Could you check a few things on this model? Use its own coordinates, in mm. A direction names the side the tool comes from. Round coordinates to 2 decimals unless told otherwise and drop trailing zeros. Loops run counter-clockwise (first coordinate to the right, second up) from the corner with the lowest first, then second, coordinate; pieces in that order, holes last. Notation, with made-up numbers: (42.25, 37.25) -> (55.25, 37.25) arc R29 cw to (55.25, 57.25) -> close; hole circle Ø2 at (66, 48.5). An arc over 180 degrees is marked (long way). One line per item, written item: value.
```python
from build123d import *

# Parameters (mm, degrees)
F1_DEPTH     = 3
F3_D         = 7
F4_W         = 24
F4_H         = 18
F5_DEPTH     = 27
F6_R         = 1.55
F7_DEPTH     = 12.5
F8_R         = 1.75
F9_DEPTH     = 12
F10_R        = 4
F11_DEPTH    = 3.4
F12_T4_DEPTH = 62
F12_T9_DEPTH = 62
F13_R        = 7
F14_T4_DEPTH = 62
F14_T9_DEPTH = 62
F15_R        = 7
F16_W        = 0.5
F16_H        = 6
F17_DEPTH    = 20
F18_R        = 5
F19_DEPTH    = 10
F20_R        = 3
F20_R_2      = 1.55
F21_DEPTH    = 3


# Not quite as in the source:
# - a fillet or chamfer that OpenCascade refuses, or shapes differently, is made with other operations: its cross-section is extruded or revolved along the edge and cut away or added


with BuildPart() as f1:
    # F0 (on Top) → F1 (new body)
    with BuildSketch(Plane.XY):
        with BuildLine():
            Line((42.5, 5), (42.5, -5))
            Line((42.5, -5), (36.1522351233, -5))
            ThreePointArc((36.1522351233, -5), (45.1458596679, -7.635020992), (50.5804776424, 0))
            ThreePointArc((50.5804776424, 0), (45.1458596679, 7.635020992), (36.1522351233, 5))
            Line((36.1522351233, 5), (42.5, 5))
        make_face()
        with BuildLine():
            ThreePointArc((-36.1522351233, 5), (-50.5804776424, 0), (-36.1522351233, -5))
            Line((-36.1522351233, -5), (-42.5, -5))
            Line((-42.5, -5), (-42.5, 5))
            Line((-42.5, 5), (-36.1522351233, 5))
        make_face()
        with BuildLine():
            Line((36.1522351233, -5), (42.5, -5))
            Line((42.5, -5), (42.5, 5))
            Line((42.5, 5), (36.1522351233, 5))
            ThreePointArc((36.1522351233, 5), (34.4195223576, 0), (36.1522351233, -5))
        make_face()
        with BuildLine():
            Line((-36.1522351233, -5), (36.1522351233, -5))
            ThreePointArc((36.1522351233, -5), (34.4195223576, 0), (36.1522351233, 5))
            Line((36.1522351233, 5), (-36.1522351233, 5))
            ThreePointArc((-36.1522351233, 5), (-34.864979008, 2.6458596679), (-34.4195223576, 0))
            ThreePointArc((-34.4195223576, 0), (-34.864979008, -2.6458596679), (-36.1522351233, -5))
        make_face()
        with BuildLine():
            Line((-42.5, -5), (-36.1522351233, -5))
            ThreePointArc((-36.1522351233, -5), (-34.864979008, -2.6458596679), (-34.4195223576, 0))
            ThreePointArc((-34.4195223576, 0), (-34.864979008, 2.6458596679), (-36.1522351233, 5))
            Line((-36.1522351233, 5), (-42.5, 5))
            Line((-42.5, 5), (-42.5, -5))
        make_face()
    extrude(amount=F1_DEPTH)

    # F3 (through all)
    with Locations(Plane.XY.offset(3)):
        with Locations((-42.5, 0), (42.5, 0)):
            Hole(F3_D / 2)

    # F4 (on Top) → F5 (join)
    with BuildSketch(Plane.XY):
        Rectangle(F4_W, F4_H)
    extrude(amount=F5_DEPTH)

    # F6 (on Front) → F7 (cut, symmetric)
    with BuildSketch(Plane.XZ):
        with Locations((0, 21.0996698588)):
            Circle(F6_R)
    extrude(amount=F7_DEPTH, both=True, mode=Mode.SUBTRACT)

    # F8 (on face) → F9 (cut)
    with BuildSketch(Plane(origin=(-12, 0, 0), x_dir=(0, -1, 0), z_dir=(-1, 0, 0))):
        with Locations((0, 21.061129868)):
            Circle(F8_R)
    extrude(amount=-F9_DEPTH, mode=Mode.SUBTRACT)

    # F10 (on face) → F11 (cut)
    with BuildSketch(Plane(origin=(-12, 0, 0), x_dir=(0, -1, 0), z_dir=(-1, 0, 0))):
        with Locations((0, 21.061129868)):
            Circle(F10_R)
    extrude(amount=-F11_DEPTH, mode=Mode.SUBTRACT)

    # F12: fillet of radius 7 on 1 edges, made by hand


with BuildPart() as f12_tool2:
    # F12_s3 → F12_t4 (new body)
    with BuildSketch(Plane.XY.offset(-17.5)):
        with BuildLine():
            ThreePointArc((-5, 9), (-9.9497474683, 6.9497474683), (-12, 2))
            Line((-12, 2), (-12, 9))
            Line((-12, 9), (-5, 9))
        make_face()
    extrude(amount=F12_T4_DEPTH)

    split(bisect_by=Plane.XZ.offset(-5), keep=Keep.BOTTOM)


with BuildPart() as f1_1:
    add(f1.part)

    # F12_t1: cut F12_tool2
    add(f12_tool2.part, mode=Mode.SUBTRACT)


with BuildPart() as f12_tool7:
    # F12_s8 → F12_t9 (new body)
    with BuildSketch(Plane.XY.offset(-17.5)):
        with BuildLine():
            ThreePointArc((-5, 9), (-9.9497474683, 6.9497474683), (-12, 2))
            Line((-12, 2), (-12, 9))
            Line((-12, 9), (-5, 9))
        make_face()
    extrude(amount=F12_T9_DEPTH)

    split(bisect_by=Plane.XY.offset(3), keep=Keep.TOP)


with BuildPart() as f1_2:
    add(f1_1.part)

    # F12_t6: cut F12_tool7
    add(f12_tool7.part, mode=Mode.SUBTRACT)

    # F13
    f13_edges = [f1_2.edges().sort_by_distance(p)[0] for p in [
        (12, 9, 13.5),
    ]]
    fillet(f13_edges, radius=F13_R)

    # F14: fillet of radius 7 on 1 edges, made by hand


with BuildPart() as f14_tool2:
    # F14_s3 → F14_t4 (new body)
    with BuildSketch(Plane.XY.offset(-17.5)):
        with BuildLine():
            ThreePointArc((-5, -9), (-9.9497474683, -6.9497474683), (-12, -2))
            Line((-12, -2), (-12, -9))
            Line((-12, -9), (-5, -9))
        make_face()
    extrude(amount=F14_T4_DEPTH)

    split(bisect_by=Plane.XZ.offset(5), keep=Keep.TOP)


with BuildPart() as f1_3:
    add(f1_2.part)

    # F14_t1: cut F14_tool2
    add(f14_tool2.part, mode=Mode.SUBTRACT)


with BuildPart() as f14_tool7:
    # F14_s8 → F14_t9 (new body)
    with BuildSketch(Plane.XY.offset(-17.5)):
        with BuildLine():
            ThreePointArc((-5, -9), (-9.9497474683, -6.9497474683), (-12, -2))
            Line((-12, -2), (-12, -9))
            Line((-12, -9), (-5, -9))
        make_face()
    extrude(amount=F14_T9_DEPTH)

    split(bisect_by=Plane.XY.offset(3), keep=Keep.TOP)


with BuildPart() as f1_4:
    add(f1_3.part)

    # F14_t6: cut F14_tool7
    add(f14_tool7.part, mode=Mode.SUBTRACT)

    # F15
    f15_edges = [f1_4.edges().sort_by_distance(p)[0] for p in [
        (12, -9, 13.5),
    ]]
    fillet(f15_edges, radius=F15_R)

    # F16 (on face) → F17 (cut)
    with BuildSketch(Plane.XY.offset(27)):
        Rectangle(F16_W, F16_H)
    extrude(amount=-F17_DEPTH, mode=Mode.SUBTRACT)

    # F18 (on face) → F19 (cut)
    with BuildSketch(Plane(origin=(0, 0, 0), x_dir=(1, 0, 0), z_dir=(0, 0, -1))):
        Circle(F18_R)
    extrude(amount=-F19_DEPTH, mode=Mode.SUBTRACT)

    # F20 (on face) → F21 (cut)
    with BuildSketch(Plane(origin=(0, 9, 0), x_dir=(-1, 0, 0), z_dir=(0, 1, 0))):
        with Locations((0, 21.0996698588)):
            Circle(F20_R)
        with Locations((0, 21.0996698588)):
            Circle(F20_R_2, mode=Mode.SUBTRACT)
    extrude(amount=-F21_DEPTH, mode=Mode.SUBTRACT)


solid = f1_4.part
```
Item 1: Will these pins go through, and if not, where does the flat tip stop? pin 1 Ø2 at (y, z) = (0, 26) entering from -X; pin 2 Ø2.5 at (x, z) = (-26.5, 1.5) entering from -Y; pin 3 Ø4.5 at (y, z) = (-0.5, 15.5) entering from +X.
Output:
pin 1: stops at x = -12
pin 2: stops at y = -5
pin 3: stops at x = 12
Item 2: If we section it at A-A on x = -42.5: List the corners of the cut face in (y, z) for me, plus the area to 3 significant figures.
Output:
outline: (-8.08, 0) -> (-3.5, 0) -> (-3.5, 3) -> (-8.08, 3) -> close; (3.5, 0) -> (8.08, 0) -> (8.08, 3) -> (3.5, 3) -> close
area: 27.5 mm²
Item 3: If we mould it in two halves opening along X, with no side actions, what happens to faces 6 (the face through (0, 9, 13)), 7 (the face through (-8.6, -2, 20)), 8 (the face through (-24, 5, 2))? For each: released by +X, released by -X, zero draft, split by the parting line, or undercut.
Output:
face 6: zero draft
face 7: released by -X
face 8: undercut
Item 4: I need wall thicknesses on line 1 (X direction, y = 0, z = 12); line 2 (X direction, y = 0.25, z = 9); line 3 (Y direction, x = -42.5, z = 1.5). Which ranges of each line are inside material? Lowest first, please. Write a range as from..to.
Output:
line 1: x = -12..-0.25, 0.25..12
line 2: x = -12..-4.99, 4.99..12
line 3: y = -8.08..-3.5, 3.5..8.08
Item 5: If we section it at C-C on x = -23: List the corners of the cut face in (y, z) for me, plus the area to 3 significant figures.
Output:
outline: (-5, 0) -> (5, 0) -> (5, 3) -> (-5, 3) -> close
area: 30.0 mm²
Item 6: For faces 1 (the face through (0.65, 7.52, 18.17)), 2 (the face through (-4.483, -1.617, 20.391)), 3 (the face through (12, 0, 15)), 4 (the face through (-0.25, 0, 25)), 5 (the face through (-12, 0, 10)), which set-ups out of +Z, -Z, +X, -X, +Y, -Y let a thin tool reach every point of the face, with its end or its side?
Output:
face 1: +Y
face 2: -X
face 3: +Z, +X, +Y, -Y
face 4: +Z, -Z
face 5: +Z, -X, +Y, -Y
Item 7: If we section it at B-B on z = 12.75: List the corners of the cut face in (x, y) for me.
Output:
outline: (-12, -2) arc R7 ccw to (-5, -9) -> (5, -9) arc R7 ccw to (12, -2) -> (12, 2) arc R7 ccw to (5, 9) -> (-5, 9) arc R7 ccw to (-12, 2) -> close; hole (-0.25, -3) -> (0.25, -3) -> (0.25, 3) -> (-0.25, 3) -> close
